CAD build for the part. Positions are in the model's coordinates, mm. A direction names the side the tool comes from. Round coordinates to 2 decimals unless told otherwise and drop trailing zeros. Order: outer loops, then holes, each group sorted by start corner. A loop starts at its lowest first (then second) coordinate and runs counter-clockwise, first axis right, second up. Notation, with made-up numbers: M 45,19.25 L 49,19.25 A31 cw 49,58.25 Z; hole C 43.25,72.25 d7. An arc over 180 degrees is marked long. Answer as CSV lines item,"result". Start each with the question number.
Autodesk Inventor part; units mm, degrees
ref_plane "YZ Plane" through (0, 0, 0) normal (1, 0, 0) x (0, 1, 0)
ref_plane "XZ Plane" through (0, 0, 0) normal (0, 1, 0) x (-1, 0, 0)
ref_plane "XY Plane" through (0, 0, 0) normal (0, 0, 1) x (1, 0, 0)
sketch "Sketch1" plane through (0, 0, 0) normal (0, 1, 0) x (-1, 0, 0)
  line L0 (21.5, 21.5) -> (-21.5, 21.5)
  line L1 (-21.5, 21.5) -> (-21.5, -21.5)
  line L2 (-21.5, -21.5) -> (21.5, -21.5)
  line L3 (21.5, -21.5) -> (21.5, 21.5)
  line L4 (21.5, 21.5) -> (-21.5, -21.5) construction
  line L5 (-21.5, 21.5) -> (21.5, -21.5) construction
  point P0 (0, 0)
  dimension "d0" = 43
  dimension "d1" = 43
extrude "Extrusion1" add sketch "Sketch1" along normal blind 10
sketch "Sketch3" plane through (0, 0, 0) normal (0, 1, 0) x (-1, 0, 0)
  line L0 (31.5, -31.5) -> (-31.5, -31.5)
  line L1 (-31.5, -31.5) -> (-31.5, 31.5)
  line L2 (-31.5, 31.5) -> (31.5, 31.5)
  line L3 (31.5, 31.5) -> (31.5, -31.5)
  line L4 (31.5, -31.5) -> (-31.5, 31.5) construction
  line L5 (-31.5, -31.5) -> (31.5, 31.5) construction
  line L6 (-21.5, 21.5) -> (-21.5, -21.5)
  line L7 (21.5, 21.5) -> (-21.5, 21.5)
  line L8 (-21.5, 21.5) -> (-21.5, -21.5)
  line L9 (-21.5, -21.5) -> (21.5, -21.5)
  line L10 (21.5, -21.5) -> (21.5, 21.5)
  line L11 (21.5, 21.5) -> (-21.5, -21.5) construction
  line L12 (-21.5, 21.5) -> (21.5, -21.5) construction
  point P0 (0, 0)
  dimension "d13" = 63
  dimension "d14" = 63
extrude "Extrusion2" add sketch "Sketch3" along normal blind 15
sketch "Sketch4" plane through (0, 15, 0) normal (0, 1, 0) x (1, 0, 0)
  line L0 (31.5, -31.5) -> (31.5, 31.5)
  line L1 (-31.5, 31.5) -> (31.5, 31.5)
  line L2 (31.5, 31.5) -> (31.5, 21.5)
  line L3 (31.5, 21.5) -> (-31.5, 21.5)
  line L4 (-31.5, 21.5) -> (-31.5, 31.5)
  point P0 (0, 0)
  dimension "d17" = 10
extrude "Extrusion3" add sketch "Sketch4" along normal blind 18
sketch "Sketch5" plane through (31.5, 0, -31.5) normal (0, 0, -1) x (-1, 0, 0)
  line L0 (0, 15) -> (0, 33) construction
  line L1 (63, 15) -> (63, 33) construction
  line L2 (0, 33) -> (63, 33) construction
  line L3 (63, 33) -> (63, 18) construction
  line L4 (63, 18) -> (0, 18) construction
  line L5 (0, 18) -> (0, 33) construction
  line L6 (0, 18) -> (0, 25.5) construction
  line L7 (0, 29.25) -> (63, 29.25)
  line L8 (63, 29.25) -> (63, 21.75)
  line L9 (63, 21.75) -> (0, 21.75)
  line L10 (-63, 29.25) -> (63, 21.75) construction
  line L11 (63, 29.25) -> (-63, 21.75) construction
  line L12 (0, 29.25) -> (0, 21.75)
  line L13 (31.5, 33) -> (31.5, 25.5) construction
  line L14 (31.5, 25.5) -> (11.5, 25.5) construction
  line L15 (31.5, 25.5) -> (51.5, 25.5) construction
  circle A0 centre (11.5, 25.5) radius 2.5
  circle A1 centre (51.5, 25.5) radius 2.5
  point P0 (31.5, 0)
  dimension "d20" = 15
  dimension "d21" = 7.5
  dimension "d22" = 7.5
  dimension "d33" = 20
  dimension "d34" = 20
  dimension "d35" = 5
  dimension "d36" = 5
sketch "Sketch6" plane through (-21.5, 10, -21.5) normal (0, 0, 1) x (1, 0, 0)
  line L0 (-10, 23) -> (53, 23) construction
  line L1 (53, 23) -> (53, 15.5) construction
  line L2 (53, -10) -> (53, 23) construction
  line L3 (53, 15.5) -> (-10, 15.5) construction
  line L4 (-10, -10) -> (-10, 23) construction
  line L5 (21.5, 23) -> (21.5, 15.5) construction
  point P0 (21.5, -10)
  dimension "d25" = 7.5
hole "Hole2" at (0, 25.5, -21.5) direction (0, 0, -1) diameter 6.1 end through all countersink diameter 11 countersink angle 90
extrude "Extrusion5" cut sketch "Sketch5" against normal blind 6 contours A0 | A1
sketch "Sketch7" plane through (0, 15, 0) normal (0, 1, 0) x (1, 0, 0)
  line L0 (-31.5, -31.5) -> (31.5, -31.5)
  line L1 (21.5, 21.5) -> (-21.5, 21.5)
  line L2 (-31.5, -31.5) -> (-21.5, -31.5)
  line L3 (-21.5, -31.5) -> (-21.5, 21.5)
  line L4 (-21.5, 21.5) -> (-31.5, 21.5)
  line L5 (-31.5, 21.5) -> (-31.5, -31.5)
  point P0 (0, 0)
extrude "Extrusion6" add sketch "Sketch7" along normal up to surface (18 mm away)
fillet "Fillet1" radius 18 1 edges at (-26.5, 33, 31.5)
sketch "Sketch9" plane through (0, 33, 0) normal (0, 1, 0) x (1, 0, 0)
  line L0 (21.5, 21.5) -> (-21.5, 21.5) construction
  line L1 (-21.5, 21.5) -> (-31.5, 21.5) construction
  line L2 (-31.5, 31.5) -> (-31.5, -13.5) construction
  line L3 (31.5, -31.5) -> (31.5, 21.5)
  line L4 (-31.5, 21.5) -> (31.5, 21.5)
  line L5 (31.5, 21.5) -> (31.5, -31.5)
  line L6 (31.5, -31.5) -> (-31.5, -31.5)
  line L7 (-31.5, -31.5) -> (-31.5, 21.5)
  point P0 (0, 0)
extrude "Extrusion7" cut sketch "Sketch9" against normal up to surface (23 mm away)
sketch "Sketch10" plane through (0, 10, 0) normal (0, 1, 0) x (1, 0, 0)
  line L0 (21.5, -21.5) -> (-21.5, -21.5)
  line L1 (-21.5, -21.5) -> (-21.5, 21.5)
  line L2 (-21.5, 21.5) -> (21.5, 21.5)
  line L3 (21.5, 21.5) -> (21.5, -21.5)
  line L4 (21.5, -21.5) -> (-21.5, 21.5) construction
  line L5 (-21.5, -21.5) -> (21.5, 21.5) construction
  line L6 (31.5, -31.5) -> (-31.5, -31.5)
  line L7 (-31.5, 31.5) -> (31.5, 31.5)
  line L8 (31.5, 31.5) -> (31.5, -31.5)
  line L9 (31.5, -31.5) -> (-31.5, -31.5)
  line L10 (-31.5, -31.5) -> (-31.5, 31.5)
  line L11 (-31.5, 31.5) -> (31.5, -31.5) construction
  line L12 (31.5, 31.5) -> (-31.5, -31.5) construction
  line L13 (-31.5, 21.5) -> (31.5, 21.5)
  line L14 (21.5, 21.5) -> (31.5, 21.5)
  line L15 (-31.5, 21.5) -> (-21.5, 21.5)
  point P0 (0, 0)
  dimension "d55" = 43
  dimension "d56" = 43
extrude "Extrusion8" cut sketch "Sketch10" against normal through all contours L3 L13 L8 L6 L10 L1 L0
fillet "Fillet2" radius 5 2 edges at (21.5, 5, -21.5) (-21.5, 5, -21.5)
sketch "Sketch11" plane through (0, 0, 0) normal (0, -1, 0) x (1, 0, 0)
  line L0 (21.5, 21.5) -> (-21.5, 21.5)
  line L1 (17, -31.5) -> (23, -31.5)
  line L2 (-21.5, 21.5) -> (21.5, 21.5)
  line L3 (21.5, 21.5) -> (21.5, -16.5)
  line L4 (21.5, -31.5) -> (-21.5, -31.5)
  line L5 (-21.5, -16.5) -> (-21.5, 21.5)
  line L6 (31.5, -21.5) -> (31.5, -31.5)
  line L7 (-26.5, -21.5) -> (-31.5, -21.5)
  line L8 (-31.5, -21.5) -> (-31.5, -31.5)
  line L9 (-31.5, -31.5) -> (31.5, -31.5)
  line L10 (31.5, -31.5) -> (31.5, -21.5)
  arc A0 (-26.5, -21.5) -> (-21.5, -16.5) centre (-26.5, -16.5) ccw
  arc A1 (21.5, -16.5) -> (26.5, -21.5) centre (26.5, -16.5) ccw
  arc A2 (21.5, -16.5) -> (26.5, -21.5) centre (26.5, -16.5) ccw
  line L11 (26.5, -21.5) -> (31.5, -21.5)
  point P0 (0, 0)
  dimension "d64" = 63
  dimension "d65" = 5
extrude "Extrusion9" add sketch "Sketch11" along normal blind 0.5
sketch "Sketch12" plane through (0, -0.5, 0) normal (0, -1, 0) x (1, 0, 0)
  line L0 (0, 0) -> (0, 10)
  line L1 (0, 0) -> (0, -10)
  dimension "d68" = 10
  dimension "d69" = 10
hole "Hole4" at (0, -0.5, -10) at (0, -0.5, 10) direction (0, 1, 0) diameter 3.1 end through all countersink diameter 5.8 countersink angle 90
properties part number "Camera Holder"
Q1. Probe line 1 along Z through (x, y) = (0, 4); line 2 along Y through (x, z) = (0, -27); line 3 along Y through (x, z) = (20, -28). List the from-to ranges inside material, lowest first. Write a range as from..to.
Q2. Drop flat-ended pins along their axis: P1, Ø2, axis at x = -2, z = -10, coming from the +Y side; P2, Ø3, axis at y = 6, z = 7, coming from the +X side; P3, Ø8, axis at x = -20, y = 25.5, coming from the +Z side; P4, Ø3, axis at x = 0, z = 10, coming from the -Y side. Give the stop position or say it passes through.
Q3. Band-saw the part on D-D, the plane x = 20. Write the cut outline in (y, z).
Q4. Band-saw the part on B-B, the plane z = -10. Write the cut outline in (x, y), then the cut area to 3 significant figures.
Q5. Tool access for faces 1 (the flat face through (0, 10, 0)), 2 (the flat face through (21.5, 5, 3)), 3 (the flat face through (0, -0.5, -5)), 4 (the flat face through (20, 26, -25.5)): list every direction of +Z, -Z, +X, -X, +Y, -Y with a clear straight run to the whole face (end or side of a thin tool).
Q6. Band-saw the part on A-A, the plane x = 0. Write the cut outline in (y, z), then the cut area to 3 significant figures.
Q7. Band-saw the part on C-C, the plane y = 25.5. Write the cut outline in (x, z), then the cut area to 3 significant figures.
Q8. Mould opens along X. For faces 5 (the flat face through (0, 33, -27)), 6 (the cylindrical face through (-18, 27, -29)), 7 (the flat face through (-21.5, 5, 2)) say: +X half, -X half, draft (parallel to the pull), parting line (faces both ways), or undercut.
Answer:
1,line 1,"z = -31.5..-11.55, -8.45..8.45, 11.55..21.5"
1,line 2,"y = -0.5..22.45, 28.55..33"
1,line 3,"y = -0.5..23, 28..33"
2,P1,"stops at y = 10"
2,P2,"stops at x = 21.5"
2,P3,"stops at z = -21.5"
2,P4,"passes through"
3,outline,"M -0.5,-31.5 L 23,-31.5 L 23,-25.5 L 28,-25.5 L 28,-31.5 L 33,-31.5 L 33,-21.5 L 10,-21.5 L 10,21.5 L -0.5,21.5 Z"
4,outline,"M -21.5,-0.5 L -2.9,-0.5 L -1.55,0.85 L -1.55,10 L -21.5,10 Z; M 1.55,0.85 L 2.9,-0.5 L 21.5,-0.5 L 21.5,10 L 1.55,10 Z"
4,area,"417 mm^2"
5,face 1,"+Z, +X, -X, +Y"
5,face 2,"+Z, +X, +Y, -Y"
5,face 3,"+Z, -Z, +X, -X, -Y"
5,face 4,"-Z"
6,outline,"M -0.5,-31.5 L 22.45,-31.5 L 22.45,-23.95 L 20,-21.5 L 10,-21.5 L 10,-11.55 L 0.85,-11.55 L -0.5,-12.9 Z; M -0.5,-7.1 L 0.85,-8.45 L 10,-8.45 L 10,8.45 L 0.85,8.45 L -0.5,7.1 Z; M -0.5,12.9 L 0.85,11.55 L 10,11.55 L 10,21.5 L -0.5,21.5 Z; M 28.55,-31.5 L 33,-31.5 L 33,-21.5 L 31,-21.5 L 28.55,-23.95 Z"
6,area,"651 mm^2"
7,outline,"M -31.5,-31.5 L -22.5,-31.5 L -22.5,-25.5 L -17.5,-25.5 L -17.5,-31.5 L -3.05,-31.5 L -3.05,-23.95 L -5.5,-21.5 L -31.5,-21.5 Z; M 3.05,-31.5 L 17.5,-31.5 L 17.5,-25.5 L 22.5,-25.5 L 22.5,-31.5 L 31.5,-31.5 L 31.5,-21.5 L 5.5,-21.5 L 3.05,-23.95 Z"
7,area,"503 mm^2"
8,face 5,"draft"
8,face 6,"undercut"
8,face 7,"-X half"
